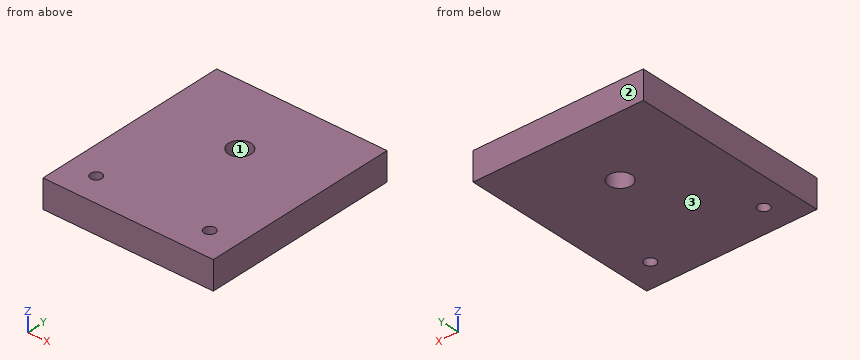
```python
from build123d import *

# Parameters (mm, degrees)
SKETCH1_W           = 60
SKETCH1_H           = 70
SKETCH1_R           = 11
SKETCH1_R_2         = 2
SKETCH1_R_3         = 4
BOSS_EXTRUDE1_DEPTH = 10


with BuildPart() as part:
    # Sketch1 → Boss-Extrude1 (new body)
    # profile 1 of 2: a face of its own
    with BuildSketch(Plane.XY):
        with Locations((0, -10)):
            Rectangle(SKETCH1_W, SKETCH1_H)
        Circle(SKETCH1_R, mode=Mode.SUBTRACT)
        with Locations((20, -35)):
            Circle(SKETCH1_R_2, mode=Mode.SUBTRACT)
        with Locations((-20, -35)):
            Circle(SKETCH1_R_2, mode=Mode.SUBTRACT)
    # profile 2 of 2: a face of its own
    with BuildSketch(Plane.XY):
        Circle(SKETCH1_R)
        Circle(SKETCH1_R_3, mode=Mode.SUBTRACT)
    extrude(amount=BOSS_EXTRUDE1_DEPTH)


solid = part.part
```
Source: CAD feature listing. Evaluate the final solid. Frame: model axes, mm. Face numbers are marked on the shaded views. Round coordinates to 2 decimals unless told otherwise and drop trailing zeros. Loops run counter-clockwise (first coordinate to the right, second up) from the corner with the lowest first, then second, coordinate; pieces in that order, holes last.
(1) Section query A-A (x = -20). Output: boundary loops of the cut face in (y, z).
From the geometry:
outline: (-45, 0) - (-37, 0) - (-37, 10) - (-45, 10) - close; (-33, 0) - (25, 0) - (25, 10) - (-33, 10) - close
(2) Pull-direction query (Y, two-part tool) for the marked faces 1, 2 and 3; classes: +Y half, -Y half, draft (parallel to the pull), parting line (faces both ways), or undercut.
From the geometry:
face 1: undercut
face 2: +Y half
face 3: draft
(3) Section query D-D (y = -35). Output: boundary loops of the cut face in (x, z), and give its area (3 significant figures).
From the geometry:
outline: (-30, 0) - (-22, 0) - (-22, 10) - (-30, 10) - close; (-18, 0) - (18, 0) - (18, 10) - (-18, 10) - close; (22, 0) - (30, 0) - (30, 10) - (22, 10) - close
area: 520 mm2
(4) Material intervals for probe 1 along Y at (x, z) = (20, 6.75); probe 2 along Y at (x, z) = (0, 5.5); probe 3 along X at (y, z) = (3, 8), sorted ascending.
From the geometry:
probe 1: y = -45 to -37, -33 to 25
probe 2: y = -45 to -4, 4 to 25
probe 3: x = -30 to -2.65, 2.65 to 30
(5) Contact query for a flat-ended pin moving along its axis: pin 1 Ø2.5 at (x, y) = (-20, -35) entering from -Z. Output: stop coordinate, or through.
From the geometry:
pin 1: passes through
(6) Section query B-B (y = 0). Output: boundary loops of the cut face in (x, z).
From the geometry:
outline: (-30, 0) - (-4, 0) - (-4, 10) - (-30, 10) - close; (4, 0) - (30, 0) - (30, 10) - (4, 10) - close
(7) Section query C-C (z = 8.25). Output: boundary loops of the cut face in (x, y), and give its area (3 significant figures).
From the geometry:
outline: (-30, -45) - (30, -45) - (30, 25) - (-30, 25) - close; hole circle Ø4 at (-20, -35); hole circle Ø8 at (0, 0); hole circle Ø4 at (20, -35)
area: 4,120 mm2
